```python
from build123d import *

# Parameters (mm, degrees)
BRACKET_BASE_DEPTH = 5
SKETCH7_R          = 5
RADIUS_1_DEPTH     = 1.5
SKETCH8_R          = 5
RADIUS_2_DEPTH     = 1.5
SKETCH9_R          = 2.5
HOLES_DEPTH        = 44.354217003


with BuildPart() as part:
    # Sketch4 → Bracket Base (new, symmetric)
    with BuildSketch(Plane(origin=(0, 0, 0), x_dir=(0, 0, -1), z_dir=(1, 0, 0))):
        with BuildLine():
            Line((1.5, 0), (1.5, 12))
            ThreePointArc((1.5, 12), (2.196870508, 15.112089987), (4.154386337, 17.629800131))
            ThreePointArc((4.154386337, 17.629800131), (6.88214507, 21.110113004), (7.898749765, 25.413572113))
            Line((7.898749765, 25.413572113), (7.898749765, 37.334358198))
            Line((7.898749765, 37.334358198), (6.398749765, 37.334358198))
            Line((6.398749765, 37.334358198), (6.398749765, 25.425719387))
            ThreePointArc((6.398749765, 25.425719387), (5.527978098, 21.755301891), (3.2, 18.787015202))
            ThreePointArc((3.2, 18.787015202), (0.840113436, 15.75178542), (0, 12))
            Line((0, 12), (0, 0))
            Line((0, 0), (1.5, 0))
        make_face()
    extrude(amount=BRACKET_BASE_DEPTH, both=True)

    # Sketch7 → Radius 1 (add)
    with BuildSketch(Plane.XY):
        Circle(SKETCH7_R)
    extrude(amount=-RADIUS_1_DEPTH)

    # Sketch8 → Radius 2 (add)
    with BuildSketch(Plane.XY.offset(-6.398749765)):
        with Locations((0, 37.334358198)):
            Circle(SKETCH8_R)
    extrude(amount=-RADIUS_2_DEPTH)

    # Sketch9 → Holes (cut, through all)
    with BuildSketch(Plane.XY):
        Circle(SKETCH9_R)
        with Locations((0, 37.334358198)):
            Circle(SKETCH9_R)
    extrude(amount=-HOLES_DEPTH, mode=Mode.SUBTRACT)


solid = part.part
```
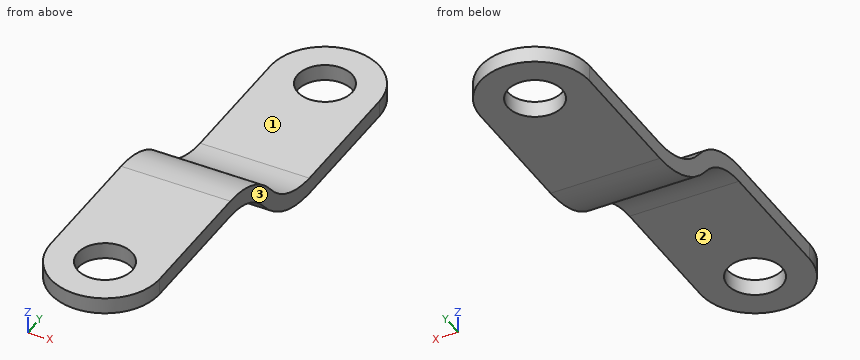
Read the model definition and answer for the solid it produces. Units are mm, in the model's axes. Face numbers are marked on the shaded views. A direction names the side the tool comes from. Coordinates: 2 decimals unless noted, no trailing zeros. Loops run counter-clockwise (first coordinate to the right, second up) from the corner with the lowest first, then second, coordinate; pieces in that order, holes last. Notation, with made-up numbers: (56, 29.5) - (101, 29.5) arc R32 cw to (101, 68.5) - close; hole circle Ø9 at (38.25, 1.25). An arc over 180 degrees is marked (long way). Answer in a Markdown table with one row per item.
1. Find section A-A, the plane x = 0. Write down the section's boundary in (y, z).
Conclusion:
| item | result |
|---|---|
| outline | (-5, -1.5) - (-2.5, -1.5) - (-2.5, 0) - (-5, 0) - close; (2.5, -1.5) - (12, -1.5) arc R7.3 cw to (17.63, -4.15) arc R10.3 ccw to (25.41, -7.9) - (34.83, -7.9) - (34.83, -6.4) - (25.43, -6.4) arc R8.8 cw to (18.79, -3.2) arc R8.8 ccw to (12, 0) - (2.5, 0) - close; (39.83, -7.9) - (42.33, -7.9) - (42.33, -6.4) - (39.83, -6.4) - close |
2. Find section C-C, the plane x = -4.25. Write down the section's boundary in (y, z).
Conclusion:
| item | result |
|---|---|
| outline | (-2.63, -1.5) - (12, -1.5) arc R7.3 cw to (17.63, -4.15) arc R10.3 ccw to (25.41, -7.9) - (39.97, -7.9) - (39.97, -6.4) - (25.43, -6.4) arc R8.8 cw to (18.79, -3.2) arc R8.8 ccw to (12, 0) - (-2.63, 0) - close |
3. Find section D-D, the plane z = -7. Write down the section's boundary in (x, y), then the cut area to 3 significant figures.
Conclusion:
| item | result |
|---|---|
| outline | (-5, 21.36) - (5, 21.36) - (5, 37.33) arc R5 ccw to (-5, 37.33) - close; hole circle Ø5 at (0, 37.33) |
| area | 179 mm² |
4. Which of the six approach directions +Z, -Z, +X, -X, +Y, -Y give full straight-line access (tool end or side, diameter ignored) to the marked faces 1, 2 and 3?
Conclusion:
| item | result |
|---|---|
| face 1 | +Z, +X, -X, +Y |
| face 2 | -Z, +X, -X, -Y |
| face 3 | +Z, -Z, +X, +Y, -Y |
5. Find section B-B, the plane y = 5.5. Write down the section's boundary in (x, z), then the cut area to 3 significant figures.
Conclusion:
| item | result |
|---|---|
| outline | (-5, -1.5) - (5, -1.5) - (5, 0) - (-5, 0) - close |
| area | 15.0 mm² |
6. Given pin 1 (5 mm diameter, centred on x = -2, y = 4.5, fed in from -Z); pin 2 (6 mm diameter, centred on x = -2.5, y = 18, fed in from +Z), each flat-ended and moving along its own axis, determine where each tip first touches the part or whether it passes through.
Conclusion:
| item | result |
|---|---|
| pin 1 | stops at z = -1.5 |
| pin 2 | stops at z = -0.53 |
7. Straight lines are drawn through the part: line 1 (Z direction, x = 0, y = 34); line 2 (Y direction, x = 0, z = -6.7); line 3 (Y direction, x = 0, z = -0.7). For each, find the intervals that lie inside material, in ascending order.
Conclusion:
| item | result |
|---|---|
| line 1 | z = -7.9 to -6.4 |
| line 2 | y = 20.75 to 34.83, 39.83 to 42.33 |
| line 3 | y = -5 to -2.5, 2.5 to 15.44 |
